Geometry check sheet. Reference: drawing and pictorial views, mm from the part's lowest x, y, z. A direction names the side the tool comes from. Round coordinates to 2 decimals unless told otherwise and drop trailing zeros. Write each loop counter-clockwise with the first axis right and the second up, starting at its lowest first coordinate (ties: lowest second). Pieces come first, ordered by that corner, then holes. Notation, with made-up numbers: M 54,46 L 88,46 A15 cw 88,62 Z; hole C 73,71 d11. An arc over 180 degrees is marked long. Answer in a Markdown table with one row per item.
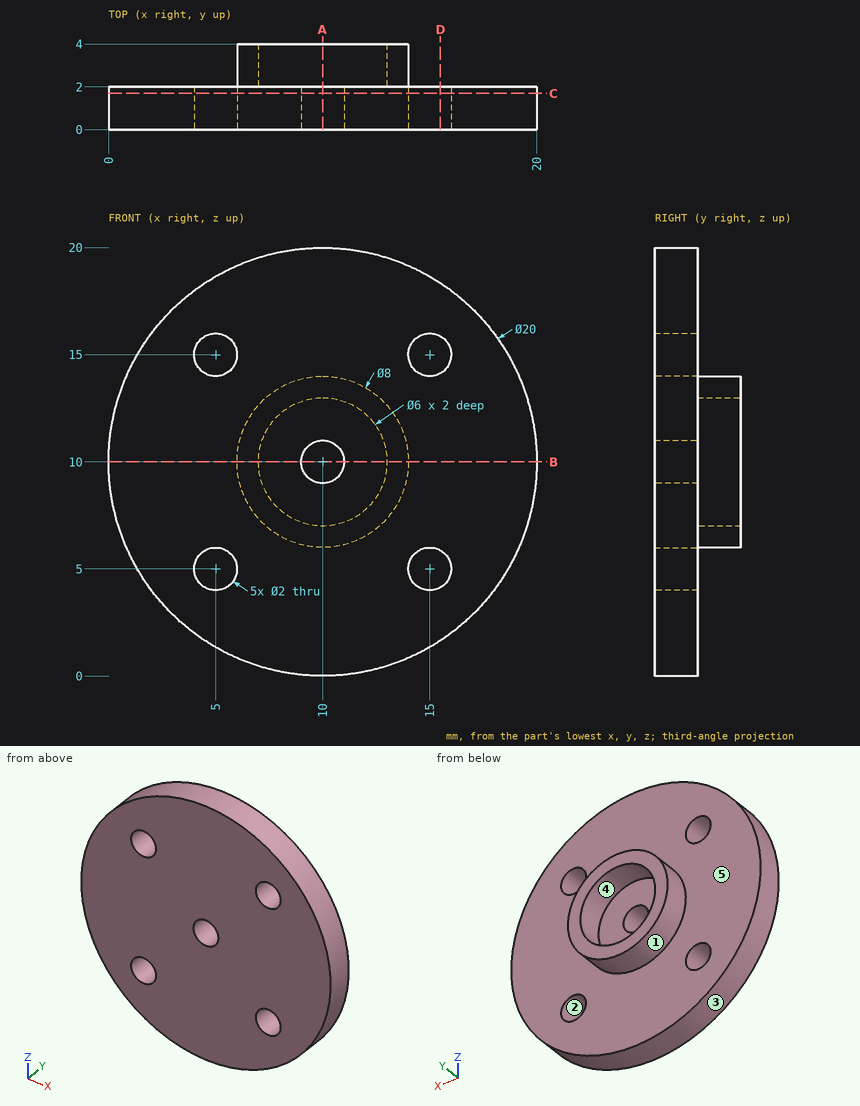
1. Section check C-C, the plane y = 1.7. Record the cut outline in (x, z), and give its area (3 significant figures).
Found:
| item | result |
|---|---|
| outline | C 10,10 d20; hole C 5,5 d2; hole C 5,15 d2; hole C 10,10 d2; hole C 15,5 d2; hole C 15,15 d2 |
| area | 298 mm2 |
2. Go/stop test with flat-tipped pins: pin 1 (1.8 mm diameter, centred on x = 9.5, z = 11, fed in from +Y); pin 2 (1.5 mm diameter, centred on x = 16, y = 0.5, fed in from +Z); pin 3 (2 mm diameter, centred on y = 2.5, z = 5, fed in from -X). Record where each tip stops, or that it passes through.
Found:
| item | result |
|---|---|
| pin 1 | stops at y = 2 |
| pin 2 | stops at z = 18.51 |
| pin 3 | stops at x = 0.89 |
3. Access from +Z, -Z, +X, -X, +Y, -Y to the whole of each face (thin tool, end or side, straight path). Record for the marked faces 1 and 2.
Found:
| item | result |
|---|---|
| face 1 | +Y |
| face 2 | +Y, -Y |
4. Draft check along X on the marked faces 3, 4 and 5. Enter one of: +X half, -X half, draft (parallel to the pull), parting line (faces both ways), or undercut.
Found:
| item | result |
|---|---|
| face 3 | parting line |
| face 4 | undercut |
| face 5 | draft |
5. Scan lines: L1, parallel to X at y = 0.75, z = 5; L2, parallel to Y at x = 6, z = 14.25; L3, parallel to X at y = 3.2, z = 10. Record each from-to range of solid material in increasing order.
Found:
| item | result |
|---|---|
| L1 | x = 1.34 to 4, 6 to 14, 16 to 18.66 |
| L2 | y = 0 to 2 |
| L3 | x = 6 to 7, 13 to 14 |
6. Section check B-B, the plane z = 10. Record the cut outline in (x, y), and give its area (3 significant figures).
Found:
| item | result |
|---|---|
| outline | M 0,0 L 9,0 L 9,2 L 7,2 L 7,4 L 6,4 L 6,2 L 0,2 Z; M 11,0 L 20,0 L 20,2 L 14,2 L 14,4 L 13,4 L 13,2 L 11,2 Z |
| area | 40.0 mm2 |
7. Section check A-A, the plane x = 10. Record the cut outline in (y, z), and give its area (3 significant figures).
Found:
| item | result |
|---|---|
| outline | M 0,0 L 2,0 L 2,6 L 4,6 L 4,7 L 2,7 L 2,9 L 0,9 Z; M 0,11 L 2,11 L 2,13 L 4,13 L 4,14 L 2,14 L 2,20 L 0,20 Z |
| area | 40.0 mm2 |
8. Section check D-D, the plane x = 15.5. Record the cut outline in (y, z), and give its area (3 significant figures).
Found:
| item | result |
|---|---|
| outline | M 0,1.65 L 2,1.65 L 2,4.13 L 0,4.13 Z; M 0,5.87 L 2,5.87 L 2,14.13 L 0,14.13 Z; M 0,15.87 L 2,15.87 L 2,18.35 L 0,18.35 Z |
| area | 26.5 mm2 |
